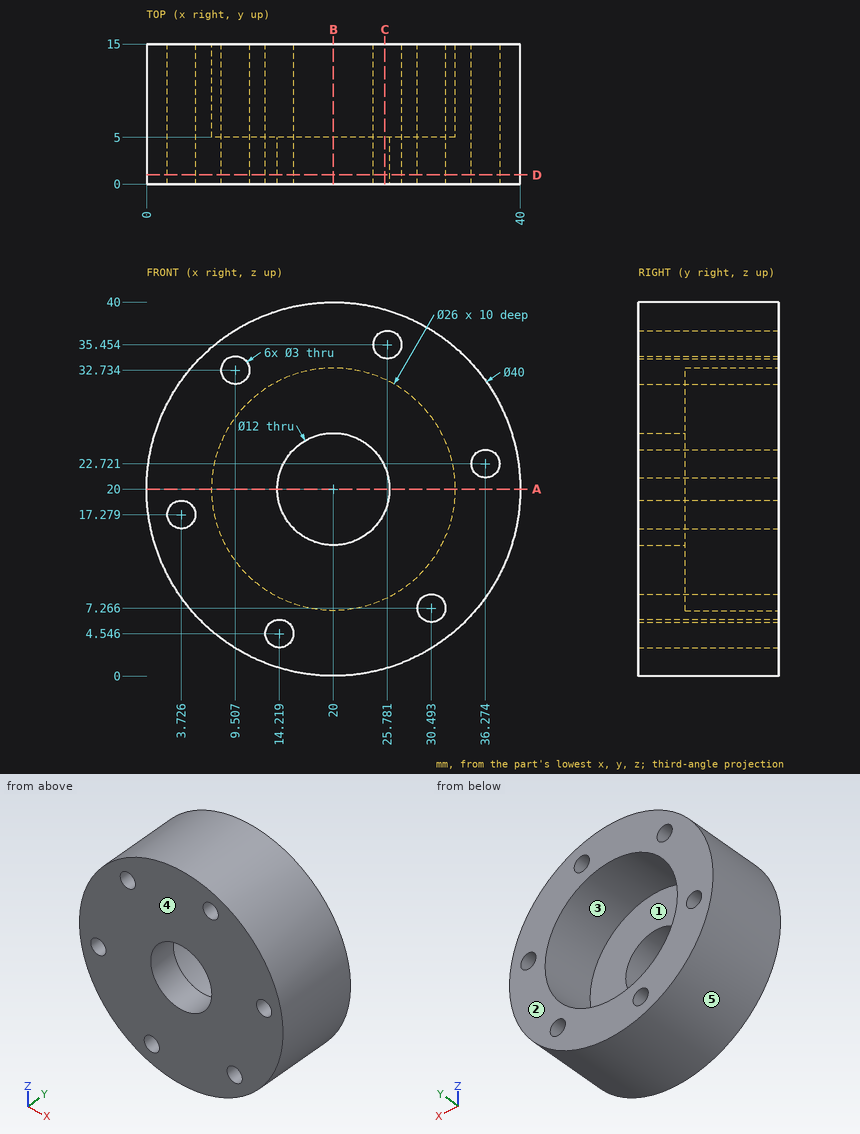
The figure shows three views and two pictorial views of one solid part (mm, origin at its lowest corner). Answer the questions. A direction names the side the tool comes from. Give positions to 0.01 mm unless a question says otherwise; leave off trailing zeros. Order: outer loops, then holes, each group sorted by start corner. A loop starts at its lowest first (then second) coordinate and runs counter-clockwise, first axis right, second up. Notation, with made-up numbers: (69, 9) -> (86, 9) arc R24 cw to (86, 23) -> close; hole circle Ø3 at (42, 54.25). An arc over 180 degrees is marked (long way). Answer as a JSON object with one key per item and string values. Group by question number.
Item 1: The part is cut by section B-B on x = 20. Write down the section's boundary in (y, z), and give its area (3 significant figures).
Item 2: The part is cut by section D-D on y = 1. Write down the section's boundary in (x, z) (1 decimal).
Item 3: The part is cut by section A-A on z = 20. Write down the section's boundary in (x, y).
Item 4: Flat-ended cylindrical pins translate along their axes: pin 1 (1.5 mm diameter, centred on y = 12.5, z = 25.5, fed in from +X); pin 2 (10 mm diameter, centred on x = 34, z = 7, fed in from -Y); pin 3 (1 mm diameter, centred on x = 10, y = 6.5, fed in from -Z); pin 4 (6 mm diameter, centred on x = 30.5, y = 7, fed in from -Z). Find the tip coordinate at first contact, or state that the pin passes through.
Item 5: A tool of negligible diameter and unlimited length cuts with its end or side. For the marked faces 1 and 2, from which of +Z, -Z, +X, -X, +Y, -Y can it reach the whole face along a straight path? Write none if from no direction.
Item 6: The part is cut by section C-C on x = 25.5. Write down the section's boundary in (y, z), and give its area (3 significant figures).
Item 7: Consider L1, parallel to X at y = 5.5, z = 16 (1 decimal); L2, parallel to Z at x = 29.5, y = 13.25 (1 decimal); L3, parallel to X at y = 1.75, z = 20. Determine where each line is inside the solid, lowest interval first. Write a range as from..to.
Item 8: Determine the mould class of the marked faces 3, 4 and 5 for opening direction Z: pulls with the +Z half, pulls with the -Z half, needs draft (parallel to the pull), parting line crosses it, or undercut.
Result set:
{
 "1": {"outline": "(0, 0) -> (15, 0) -> (15, 7) -> (5, 7) -> (5, 14) -> (0, 14) -> close; (0, 26) -> (5, 26) -> (5, 33) -> (15, 33) -> (15, 40) -> (0, 40) -> close", "area": "280 mm²"},
 "2": {"outline": "circle Ø40 at (20, 20); hole circle Ø3 at (3.7, 17.3); hole circle Ø3 at (9.5, 32.7); hole circle Ø3 at (14.2, 4.5); hole circle Ø12 at (20, 20); hole circle Ø3 at (25.8, 35.5); hole circle Ø3 at (30.5, 7.3); hole circle Ø3 at (36.3, 22.7)"},
 "3": {"outline": "(0, 0) -> (14, 0) -> (14, 5) -> (7, 5) -> (7, 15) -> (0, 15) -> close; (26, 0) -> (40, 0) -> (40, 15) -> (33, 15) -> (33, 5) -> (26, 5) -> close"},
 "4": {"pin 1": "x = 39.43", "pin 2": "y = 0", "pin 3": "z = 2.4", "pin 4": "z = 1.46"},
 "5": {"face 1": "+Y", "face 2": "+Z, -Z, +X, -X, +Y"},
 "6": {"outline": "(0, 0.77) -> (15, 0.77) -> (15, 8.22) -> (5, 8.22) -> (5, 17.6) -> (0, 17.6) -> close; (0, 22.4) -> (5, 22.4) -> (5, 31.78) -> (15, 31.78) -> (15, 33.98) -> (0, 33.98) -> close; (0, 36.93) -> (15, 36.93) -> (15, 39.23) -> (0, 39.23) -> close", "area": "273 mm²"},
 "7": {"L1": "0.4..2.9, 4.5..7.6, 32.4..39.6", "L2": "2.4..6.1, 8.4..11.1, 28.9..37.6", "L3": "0..14, 26..40"},
 "8": {"face 3": "undercut", "face 4": "needs draft", "face 5": "parting line crosses it"}
}
